Check sheet for the modelled part. Datum: model origin and axes. Units: mm. A direction names the side the tool comes from. Give positions to 0.01 mm unless a question says otherwise; leave off trailing zeros. Loops run counter-clockwise (first coordinate to the right, second up) from the corner with the lowest first, then second, coordinate; pieces in that order, holes last. Notation, with made-up numbers: M 50.5,70 L 82.5,70 A36 ccw 82.5,107 Z; hole C -9.75,-2 d7. An arc over 180 degrees is marked long. Put each result on its own line as item: value. Start each with the question number.
```python
from build123d import *

# Parameters (mm, degrees)
BOSS_EXTRUDE5_DEPTH = 150
CUT_EXTRUDE4_DEPTH  = 130
SKETCH8_R           = 47.5
CUT_EXTRUDE5_DEPTH  = 475.65402898


with BuildPart() as part:
    # Sketch1 → Boss-Extrude5 (new body)
    with BuildSketch(Plane(origin=(0, 0, 0), x_dir=(1, 0, 0), z_dir=(0, 1, 0))):
        with BuildLine():
            Line((-180, 150), (180, 150))
            ThreePointArc((180, 150), (194.142135624, 144.142135624), (200, 130))
            Line((200, 130), (200, -137.480797285))
            ThreePointArc((200, -137.480797285), (196.889858076, -148.19213213), (188.526730584, -155.572089819))
            add(Edge.make_bspline(
                [(-188.526730584, -155.572089819), (-94.263365292, -200), (0, -244.427910181), (188.526730584, -155.572089819)],
                knots=[0, 0, 0, 0, 1, 1, 1, 1], degree=3))
            ThreePointArc((-188.526730584, -155.572089819), (-196.889858076, -148.19213213), (-200, -137.480797285))
            Line((-200, -137.480797285), (-200, 130))
            ThreePointArc((-200, 130), (-194.142135624, 144.142135624), (-180, 150))
        make_face()
    extrude(amount=BOSS_EXTRUDE5_DEPTH)

    # Sketch7 → Cut-Extrude4 (cut)
    with BuildSketch(Plane.XZ):
        with BuildLine():
            Line((-180, -135), (180, -135))
            ThreePointArc((180, -135), (183.535533906, -133.535533906), (185, -130))
            Line((185, -130), (185, 137.480797285))
            ThreePointArc((185, 137.480797285), (184.222464519, 140.158630996), (182.131682646, 142.003620419))
            add(Edge.make_bspline(
                [(182.131682646, 142.003620419), (167.754395175, 148.779877923), (153.243793404, 155.096016084), (123.887544981, 166.571922609), (109.042273823, 171.732986949), (86.451364448, 178.35977611), (78.866974419, 180.382030951), (63.574333937, 183.999050287), (55.866097219, 185.593862184), (40.307101742, 188.29158715), (32.456347746, 189.394516661), (20.556839665, 190.62308876), (16.569747475, 190.961550457), (8.551333739, 191.485821191), (4.544231323, 191.669927655), (-7.454411488, 191.980616602), (-15.430189587, 191.865523988), (-31.333284121, 190.965648075), (-39.260577272, 190.180543026), (-51.114854999, 188.496254108), (-55.060184136, 187.85057332), (-60.969143231, 186.757203044), (-62.937291634, 186.371953854), (-66.870612209, 185.560327), (-68.836067076, 185.13383579), (-78.618097665, 182.909176108), (-86.329542172, 180.827443766), (-101.559170643, 176.152807331), (-109.077405353, 173.560037463), (-123.963089417, 167.97567232), (-131.330609371, 164.984263785), (-153.278917059, 155.602043077), (-167.705359418, 148.8029893), (-182.131682646, 142.003620419)],
                knots=[0, 0, 0, 0, 0.125, 0.125, 0.25, 0.25, 0.3125, 0.3125, 0.375, 0.375, 0.4375, 0.4375, 0.46875, 0.46875, 0.5, 0.5, 0.5625, 0.5625, 0.625, 0.625, 0.65625, 0.65625, 0.671875, 0.671875, 0.6875, 0.6875, 0.75, 0.75, 0.8125, 0.8125, 0.875, 0.875, 1, 1, 1, 1], degree=3))
            ThreePointArc((-182.131682646, 142.003620419), (-184.222464519, 140.158630996), (-185, 137.480797285))
            Line((-185, 137.480797285), (-185, -130))
            ThreePointArc((-185, -130), (-183.535533906, -133.535533906), (-180, -135))
        make_face()
    extrude(amount=-CUT_EXTRUDE4_DEPTH, mode=Mode.SUBTRACT)

    # Sketch8 → Cut-Extrude5 (cut, through all)
    with BuildSketch(Plane(origin=(200, 0, 0), x_dir=(0, 0, -1), z_dir=(1, 0, 0))):
        with Locations((-2.574719222, 2.5)):
            Circle(SKETCH8_R)
    extrude(amount=-CUT_EXTRUDE5_DEPTH, mode=Mode.SUBTRACT)


solid = part.part
```
Q1. Section check A-A, the plane z = -86. Record the cut outline in (x, y), then the cut area to 3 significant figures.
Q2. Mould release check, pull along Z, two halves, no side actions. Record for faces 1 (the face through (-196.8, 73.95, 148.33)), 2 (the face through (1, 0, -137)), 3 (the face through (192.605, 49.988, 1.495)), 4 (the face through (185, 64, 2)): pulls with the +Z half, pulls with the -Z half, needs draft (parallel to the pull), parting line crosses it, or undercut.
Q3. Depth check by flat-ended pin: P1, Ø2, axis at x = -66, z = -1, coming from the -Y side. Enter the tip coordinate at first touch or a pass-through.
Q4. Access from +Z, -Z, +X, -X, +Y, -Y to the whole of each face (thin tool, end or side, straight path). Record for faces 5 (the face through (-3, 130, 31)), 6 (the face through (-200, 74, 6)).
Q5. Section check B-B, the plane z = 33. Record the cut outline in (x, y), then the cut area to 3 significant figures.
Q6. Thickness scan on line 1 along X through (y, z) = (64, -82.5); line 2 along Y through (x, z) = (162, 146.5); line 3 along Z through (x, y) = (-163, 55). Record the ranges inside material, lowest first. Write a range as [from, to].
Found:
1. outline: M -200,0 L -185,0 L -185,130 L 185,130 L 185,0 L 200,0 L 200,150 L -200,150 Z
1. area: 11,900 mm^2
2. face 1: pulls with the +Z half
2. face 2: needs draft
2. face 3: undercut
2. face 4: undercut
3. P1: stops at y = 130
4. face 5: -Y
4. face 6: +Z, -Z, -X, +Y, -Y
5. outline: M -200,38.98 L -185,38.98 L -185,130 L 185,130 L 185,38.98 L 200,38.98 L 200,150 L -200,150 Z
5. area: 10,700 mm^2
6. line 1: x = [-200, -185], [185, 200]
6. line 2: y = [130, 150]
6. line 3: z = [-150, -135], [150.97, 167.47]
